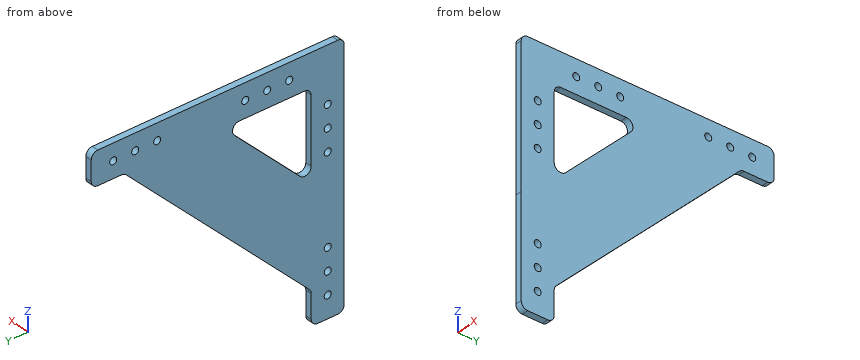
Autodesk Inventor part; units mm, degrees
ref_plane "YZ Plane" through (0, 0, 0) normal (1, 0, 0) x (0, 1, 0)
ref_plane "XZ Plane" through (0, 0, 0) normal (0, 1, 0) x (-1, 0, 0)
ref_plane "XY Plane" through (0, 0, 0) normal (0, 0, 1) x (1, 0, 0)
sketch "スケッチ1" plane through (0, 0, 0) normal (1, 0, 0) x (0, 1, 0)
  line L0 (0, 0) -> (0, -115)
  line L1 (0, 0) -> (115, 0) construction
  line L2 (0, 0) -> (115, 0)
  line L3 (0, 0) -> (115, 0) construction
  line L4 (115, 0) -> (0, -115)
  dimension "d0" = 115
  dimension "d1" = 90
  dimension "d2" = 115
  dimension "d3" = 0
extrude "押し出し1" add sketch "スケッチ1" along normal blind 3
sketch "スケッチ2" plane through (3, 0, 0) normal (1, 0, 0) x (0, 0, -1)
  line L0 (0, 0) -> (0, 65)
  line L1 (0, 115) -> (0, 0)
  line L2 (0, 0) -> (65, 0) construction
  line L3 (0, 0) -> (65, 0)
  line L4 (0, 0) -> (115, 0)
  line L5 (0, 0) -> (65, 0) construction
  line L6 (65, 0) -> (0, 65)
  dimension "d6" = 65
  dimension "d7" = 90
  dimension "d8" = 65
  dimension "d9" = 0
extrude "押し出し2" cut sketch "スケッチ2" against normal blind 3
sketch "スケッチ3" plane through (3, 0, 0) normal (1, 0, 0) x (0, 0, -1)
  line L0 (0, 115) -> (15, 115)
  line L1 (0, 115) -> (15, 115) construction
  line L2 (15, 115) -> (15, 100)
  line L3 (115, 0) -> (0, 115)
  line L4 (115, 0) -> (115, 15)
  line L5 (115, 0) -> (130, 0) construction
  line L6 (115, 15) -> (100, 15)
  point P0 (0, 0)
  dimension "d12" = 15
  dimension "d13" = 0
  dimension "d14" = 15
  dimension "d15" = 90
extrude "押し出し3" add sketch "スケッチ3" against normal blind 3
sketch "スケッチ4" plane through (3, 0, 0) normal (1, 0, 0) x (0, 0, -1)
  line L0 (15, 115) -> (0, 115)
  line L1 (15, 100) -> (15, 115)
  line L2 (0, 115) -> (0, 65)
  line L3 (0, 0) -> (95, 95) construction
  line L4 (0, 0) -> (134.3503, 0) construction
  point P0 (7.5, 105)
  point P1 (7.5, 95)
  point P2 (7.5, 85)
  point P3 (105, 7.5)
  point P4 (95, 7.5)
  point P5 (85, 7.5)
  dimension "d18" = 10
  dimension "d19" = 7.5
  dimension "d20" = 7.5
  dimension "d21" = 7.5
  dimension "d22" = 10
  dimension "d23" = 10
  dimension "d24" = 45
hole "穴1" at (3, 105, -7.5) at (3, 95, -7.5) at (3, 85, -7.5) at (3, 7.5, -105) at (3, 7.5, -95) at (3, 7.5, -85) direction (-1, 0, 0) diameter 3.2 end through all
fillet "フィレット1" radius 3 8 edges at (1.5, 115, -15) (1.5, 100, -15) (1.5, 15, -100) (1.5, 15, -115) (1.5, 0, -115) (1.5, 0, -65) (1.5, 65, 0) (1.5, 115, 0)
sketch "スケッチ5" plane through (3, 0, 0) normal (1, 0, 0) x (0, 0, -1)
  line L0 (0, 0) -> (65, 0)
  line L1 (66.2426, 0) -> (112, 0)
  line L2 (0, 0) -> (66.2426, 0)
  arc A0 (0, 66.2426) -> (0.8787, 64.1213) centre (3, 66.2426) ccw
  line L3 (0, 0) -> (0, 66.2426)
  line L4 (0.8787, 64.1213) -> (64.1213, 0.8787)
  line L5 (0.8787, 64.1213) -> (64.1213, 0.8787)
  arc A1 (0, 66.2426) -> (0.8787, 64.1213) centre (3, 66.2426) ccw
  arc A2 (64.1213, 0.8787) -> (66.2426, 0) centre (66.2426, 3) ccw
extrude "押し出し4" add sketch "スケッチ5" against normal blind 3
sketch "スケッチ6" plane through (3, 0, 0) normal (1, 0, 0) x (0, 0, -1)
  line L0 (0, 0) -> (112, 0)
  line L1 (0, 112) -> (0, 0)
  line L2 (15, 15) -> (55, 15)
  line L3 (55, 15) -> (15, 55)
  line L4 (15, 55) -> (15, 15)
  dimension "d35" = 15
  dimension "d36" = 15
  dimension "d37" = 40
  dimension "d38" = 40
extrude "押し出し5" cut sketch "スケッチ6" against normal blind 3
sketch "スケッチ7" plane through (3, 0, 0) normal (1, 0, 0) x (0, 0, -1)
  line L0 (0, 112) -> (0, 0)
  line L1 (0, 0) -> (112, 0)
  line L2 (0, 0) -> (0, 112)
  line L3 (0, 0) -> (76.3955, 76.3955) construction
  line L4 (0, 0) -> (108.0395, 0) construction
  point P0 (7.5, 25)
  point P1 (7.5, 35)
  point P2 (7.5, 45)
  point P3 (25, 7.5)
  point P4 (35, 7.5)
  point P5 (45, 7.5)
  dimension "d41" = 7.5
  dimension "d42" = 25
  dimension "d43" = 10
  dimension "d44" = 10
  dimension "d46" = 45
hole "穴2" at (3, 25, -7.5) at (3, 35, -7.5) at (3, 45, -7.5) at (3, 7.5, -25) at (3, 7.5, -35) at (3, 7.5, -45) direction (-1, 0, 0) diameter 3.2 end through all
fillet "フィレット2" radius 3 4 edges at (1.5, 15, -55) (1.5, 55, -15) (1.5, 15, -15) (1.5, 0, 0)
properties part number "射出_固定2" material "アルミニウム 6061"
Here's how the part is built. I have some questions about the finished solid (model axes, mm). Round coordinates to 2 decimals unless told otherwise and drop trailing zeros. Write each loop counter-clockwise with the first axis right and the second up, starting at its lowest first coordinate (ties: lowest second). Pieces come first, ordered by that corner, then holes. Notation, with made-up numbers: M -35.75,-18.5 L -4.75,-18.5 A28 ccw -4.75,18.5 Z; hole C 69.25,-32.75 d2. An arc over 180 degrees is marked long. Answer as CSV lines item,"result". Start each with the question number.
1. Suppose I cut it at D-D on z = -85. Write out the boundary of the cut face in (x, y).
2. Suppose I cut it at C-C on y = 45. Write out the boundary of the cut face in (x, z), then the cut area to 3 significant figures.
3. I'm going to push flat-ended pins straight in: pin 1 Ø1.9 at (y, z) = (85, -7.5) entering from +X; pin 2 Ø1.5 at (x, y) = (1, 29) entering from -Z; pin 3 Ø1.5 at (x, y) = (1.5, 109.5) entering from -Z. Where does each tip first touch, or does it pass through?
4. Suppose I cut it at A-A on z = -45. Write out the boundary of the cut face in (x, y).
5. Suppose I cut it at B-B on x = 2.45. Count the separate pieces of the cut face and the enclosed holes in it, then the cut area to 3 significant figures.
6. I need wall thicknesses on probe 1 along Y at (x, z) = (1.9, -37); probe 2 along Z at (x, y) = (1.15, 32.5); probe 3 along Z at (x, y) = (2.1, 85). Which ranges of each line are inside material? Lowest first, please.
Check result:
1,outline,"M 0,0 L 3,0 L 3,5.9 L 0,5.9 Z; M 0,9.1 L 3,9.1 L 3,30 L 0,30 Z"
2,outline,"M 0,-70 L 3,-70 L 3,-25 L 0,-25 Z; M 0,-15 L 3,-15 L 3,-9.1 L 0,-9.1 Z; M 0,-5.9 L 3,-5.9 L 3,0 L 0,0 Z"
2,area,"170 mm2"
3,pin 1,"passes through"
3,pin 2,"stops at z = -86.75"
3,pin 3,"stops at z = -15"
4,outline,"M 0,0 L 3,0 L 3,5.9 L 0,5.9 Z; M 0,9.1 L 3,9.1 L 3,15 L 0,15 Z; M 0,25 L 3,25 L 3,70 L 0,70 Z"
5,separate pieces,"1"
5,enclosed holes,"13"
5,area,"5,960 mm2"
6,probe 1,"y = 0 to 15, 33 to 78"
6,probe 2,"z = -82.5 to -37.5, -15 to 0"
6,probe 3,"z = -30 to -9.1, -5.9 to 0"
